For this review, take the finished solid that the model builds, in its own axes (mm). Face numbers are marked on the shaded views. A direction names the side the tool comes from. Coordinates: 2 decimals unless noted, no trailing zeros. Loops run counter-clockwise (first coordinate to the right, second up) from the corner with the lowest first, then second, coordinate; pieces in that order, holes last. Notation, with made-up numbers: (-29, -2.5) -> (10, -2.5) arc R9 ccw to (10, 8.5) -> close; hole circle Ø7 at (-26.5, 71.5). An arc over 180 degrees is marked (long way). One line per item, written item: value.
from build123d import *

# Parameters (mm, degrees)
CROQUIS1_W              = 150
CROQUIS1_H              = 40
SALIENTE_EXTRUIR1_DEPTH = 25.4
CORTAR_EXTRUIR1_DEPTH   = 82.671047502
CHAFL_N1_SIZE           = 5
CHAFL_N2_SIZE           = 3
CORTAR_EXTRUIR2_DEPTH   = 82.671047502
CROQUIS5_R              = 2.75
CORTAR_EXTRUIR3_DEPTH   = 16
CROQUIS6_R              = 2.75
CORTAR_EXTRUIR4_DEPTH   = 16
CORTAR_EXTRUIR8_START   = -16
CROQUIS7_R              = 2.75
CORTAR_EXTRUIR8_DEPTH   = 16
CROQUIS8_R              = 2.75
CORTAR_EXTRUIR9_DEPTH   = 16


with BuildPart() as part:
    # Croquis1 → Saliente-Extruir1 (new body)
    with BuildSketch(Plane(origin=(0, 0, 0), x_dir=(1, 0, 0), z_dir=(0, 1, 0))):
        Rectangle(CROQUIS1_W, CROQUIS1_H)
    extrude(amount=SALIENTE_EXTRUIR1_DEPTH)

    # Croquis2 → Cortar-Extruir1 (cut, through all)
    with BuildSketch(Plane(origin=(0, 25.4, 0), x_dir=(1, 0, 0), z_dir=(0, 1, 0))):
        Polygon((-42, 20), (-42, 17), (61, 17), (61, 19), (75, 19), (75, 20), (60, 20), align=None)
        Polygon((43, -20), (43, -17), (-41, -17), (-41, -19), (-75, -19), (-75, -20), align=None)
    extrude(amount=-CORTAR_EXTRUIR1_DEPTH, mode=Mode.SUBTRACT)

    # Chaflán1
    # the kernel refuses this chamfer: 5 mm, written as the material it adds along each edge
    with BuildSketch(Plane(origin=(43, 25.4, 17), x_dir=(-0.9996219169112968, 0, -0.027495876610586317), z_dir=(0, -1, 0))) as chafl_n1_piece_1_section:
        Polygon((CHAFL_N1_SIZE * 0.999621916911, -CHAFL_N1_SIZE * 0.0274958766106), (-CHAFL_N1_SIZE * 0.0274958766106, -CHAFL_N1_SIZE * 0.999621916911), (0, 0), align=None)
    chafl_n1_piece_1 = extrude(amount=25.4, mode=Mode.PRIVATE)
    chafl_n1_piece_1 = split(chafl_n1_piece_1, bisect_by=Plane(origin=(41.124952702, 12.7, 20), z_dir=(0, 0, -1)), keep=Keep.TOP, mode=Mode.PRIVATE)
    add(chafl_n1_piece_1)
    with BuildSketch(Plane(origin=(-42, 25.4, -17), x_dir=(-0.027495876610586317, 0, -0.9996219169112968), z_dir=(0, -1, 0))) as chafl_n1_piece_2_section:
        Polygon((CHAFL_N1_SIZE * 0.999621916911, CHAFL_N1_SIZE * 0.0274958766106), (-CHAFL_N1_SIZE * 0.0274958766106, CHAFL_N1_SIZE * 0.999621916911), (0, 0), align=None)
    chafl_n1_piece_2 = extrude(amount=25.4, mode=Mode.PRIVATE)
    chafl_n1_piece_2 = split(chafl_n1_piece_2, bisect_by=Plane(origin=(-40.124952702, 12.7, -20), z_dir=(0, 0, 1)), keep=Keep.TOP, mode=Mode.PRIVATE)
    add(chafl_n1_piece_2)

    # Chaflán2
    # the kernel refuses this chamfer: 3 mm, written as the material it adds along each edge
    with BuildSketch(Plane(origin=(-41, 25.4, 17), x_dir=(-0.027495876610586768, 0, 0.9996219169112968), z_dir=(0, -1, 0))) as chafl_n2_piece_1_section:
        Polygon((CHAFL_N2_SIZE * 0.999621916911, -CHAFL_N2_SIZE * 0.0274958766106), (-CHAFL_N2_SIZE * 0.0274958766106, -CHAFL_N2_SIZE * 0.999621916911), (0, 0), align=None)
    chafl_n2_piece_1 = extrude(amount=25.4, mode=Mode.PRIVATE)
    chafl_n2_piece_1 = split(chafl_n2_piece_1, bisect_by=Plane(origin=(-39.907908995, 12.7, 19), z_dir=(0, 0, -1)), keep=Keep.TOP, mode=Mode.PRIVATE)
    add(chafl_n2_piece_1)
    with BuildSketch(Plane(origin=(61, 25.4, -17), x_dir=(0.027495876610586768, 0, -0.9996219169112968), z_dir=(0, -1, 0))) as chafl_n2_piece_2_section:
        Polygon((CHAFL_N2_SIZE * 0.999621916911, -CHAFL_N2_SIZE * 0.0274958766106), (-CHAFL_N2_SIZE * 0.0274958766106, -CHAFL_N2_SIZE * 0.999621916911), (0, 0), align=None)
    chafl_n2_piece_2 = extrude(amount=25.4, mode=Mode.PRIVATE)
    chafl_n2_piece_2 = split(chafl_n2_piece_2, bisect_by=Plane(origin=(59.907908995, 12.7, -19), z_dir=(0, 0, 1)), keep=Keep.TOP, mode=Mode.PRIVATE)
    add(chafl_n2_piece_2)

    # Croquis3 → Cortar-Extruir2 (cut, through all)
    with BuildSketch(Plane(origin=(0, 25.4, 0), x_dir=(1, 0, 0), z_dir=(0, 1, 0))):
        with BuildLine():
            Line((-15, 8), (-5, 8))
            ThreePointArc((-5, 8), (3, 16), (11, 8))
            Line((11, 8), (11, -9.5))
            ThreePointArc((11, -9.5), (3, -16.34938703), (-5, -9.5))
            Line((-5, -9.5), (-15, -9.5))
            ThreePointArc((-15, -9.5), (-23, -16.349387053), (-31, -9.5))
            Line((-31, -9.5), (-31, 8))
            ThreePointArc((-31, 8), (-23, 16), (-15, 8))
        make_face()
    extrude(amount=-CORTAR_EXTRUIR2_DEPTH, mode=Mode.SUBTRACT)

    # Croquis5 → Cortar-Extruir3 (cut)
    with BuildSketch(Plane(origin=(0, 0, -20), x_dir=(-1, 0, 0), z_dir=(0, 0, -1))):
        with Locations((68.9, 12.7)):
            Circle(CROQUIS5_R)
        with Locations((49.8, 12.7)):
            Circle(CROQUIS5_R)
    extrude(amount=-CORTAR_EXTRUIR3_DEPTH, mode=Mode.SUBTRACT)

    # Croquis6 → Cortar-Extruir4 (cut)
    with BuildSketch(Plane.ZY.offset(75)):
        with Locations((9.05, 12.7)):
            Circle(CROQUIS6_R)
        with Locations((-10.05, 12.7)):
            Circle(CROQUIS6_R)
    extrude(amount=-CORTAR_EXTRUIR4_DEPTH, mode=Mode.SUBTRACT)

    # Croquis7 → Cortar-Extruir8 (cut)
    with BuildSketch(Plane.XY.offset(19).offset(CORTAR_EXTRUIR8_START)):
        with Locations(Location((-68.9, 12.7, 0), (0, 0, 180))):
            Circle(CROQUIS7_R)
        with Locations(Location((-49.8, 12.7, 0), (0, 0, 180))):
            Circle(CROQUIS7_R)
    extrude(amount=CORTAR_EXTRUIR8_DEPTH, mode=Mode.SUBTRACT)

    # Croquis8 → Cortar-Extruir9 (cut)
    with BuildSketch(Plane.XY.offset(20)):
        with Locations((49.8, 12.7)):
            Circle(CROQUIS8_R)
        with Locations((68.9, 12.7)):
            Circle(CROQUIS8_R)
    extrude(amount=-CORTAR_EXTRUIR9_DEPTH, mode=Mode.SUBTRACT)


solid = part.part
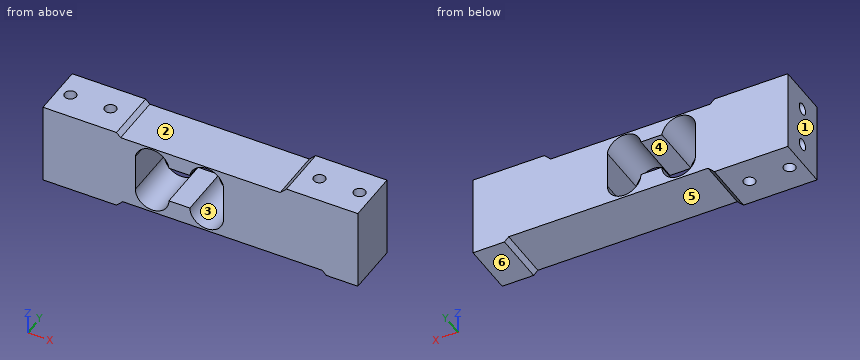
1. Take a section at C-C, the plane y = 23.5. Give the boundary of the cut face in (x, z).
Return value:
outline: (-75, -20) -> (-40, -20) -> (-37, -17) -> (58, -17) -> (60, -19) -> (75, -19) -> (75, 20) -> (41, 20) -> (38, 17) -> (-38, 17) -> (-40, 19) -> (-75, 19) -> close; hole (-31, -8) arc R8 ccw to (-15, -8) -> (-5, -8) arc R8 ccw to (11, -8) -> (11, 9.5) arc R8.1 ccw to (-5, 9.5) -> (-15, 9.5) arc R8.1 ccw to (-31, 9.5) -> close
2. Take a section at B-B, the plane x = -23. Give the boundary of the cut face in (y, z).
Return value:
outline: (0, -17) -> (25.4, -17) -> (25.4, -16) -> (0, -16) -> close; (0, 16.35) -> (25.4, 16.35) -> (25.4, 17) -> (0, 17) -> close
3. For the marked faces 4, 5 and 6, list the 3-axis set-ups (+Z, -Z, +X, -X, +Y, -Y) from which the entire face can be reached by the end or side of a thin tool; tool diameter is ignored.
Return value:
face 4: +Y, -Y
face 5: -Z, +Y, -Y
face 6: -Z, +X, +Y, -Y
4. Take a section at A-A, the plane z = 0. Give the boundary of the cut face in (x, y), and give its area (3 significant figures).
Return value:
outline: (-75, 0) -> (-31, 0) -> (-31, 25.4) -> (-75, 25.4) -> close; (11, 0) -> (75, 0) -> (75, 25.4) -> (11, 25.4) -> close
area: 2,740 mm2
5. Insertion check: pin 1 Ø8 at (x, y) = (42, 5) entering from -Z; pin 2 Ø1.6 at (x, y) = (-68.5, 13) entering from -Z; pin 3 Ø5 at (x, y) = (-12.5, 18) entering from +Z. Each pin has a flat end and moves straight along its axis. Give the tip position at first contact, or say it passes through.
Return value:
pin 1: stops at z = -17
pin 2: stops at z = -4
pin 3: stops at z = 17
6. The part is to be moulded in two halves that separate along Z. For the marked faces 1, 2 and 3, say which applies: pulls with the +Z half, pulls with the -Z half, needs draft (parallel to the pull), parting line crosses it, or undercut.
Return value:
face 1: needs draft
face 2: pulls with the +Z half
face 3: undercut
7. To check wall thickness, follow probe 1 along Z at (x, y) = (-62.75, 12.7); probe 2 along X at (y, z) = (20.75, 4.5); probe 3 along Y at (x, z) = (-65, 9). State the ranges of each line that lie inside material, in increasing order. Write a range as from..to.
Return value:
probe 1: z = -20..-12.8, -7.3..6.3, 11.8..19
probe 2: x = -75..-31, 11..75
probe 3: y = 0..9.95, 15.45..25.4
8. Take a section at D-D, the plane x = -49.8. Give the boundary of the cut face in (y, z).
Return value:
outline: (0, -20) -> (9.95, -20) -> (9.95, -4) -> (15.45, -4) -> (15.45, -20) -> (25.4, -20) -> (25.4, 19) -> (15.45, 19) -> (15.45, 3) -> (9.95, 3) -> (9.95, 19) -> (0, 19) -> close
